Autodesk Inventor part; units mm, degrees
ref_plane "YZ Plane" through (0, 0, 0) normal (1, 0, 0) x (0, 1, 0)
ref_plane "XZ Plane" through (0, 0, 0) normal (0, 1, 0) x (-1, 0, 0)
ref_plane "XY Plane" through (0, 0, 0) normal (0, 0, 1) x (1, 0, 0)
sketch "Skizze1" plane through (0, 0, 0) normal (0, 1, 0) x (-1, 0, 0)
  circle A0 centre (32.7504, -19.9257) radius 25
  line L0 (32.7504, -19.9257) -> (-77.2496, -19.9257)
  line L1 (-77.2496, -19.9257) -> (-77.2496, -22.4257)
  line L2 (-77.2496, -22.4257) -> (7.8757, -22.4257)
  line L3 (7.8757, -22.4257) -> (7.8757, -19.9257)
  point P0 (0, 0)
  dimension "d4" = 50
  dimension "d9" = 110
  dimension "d10" = 2.5
extrude "Extrusion1" add sketch "Skizze1" along normal blind 1.5 and the other way blind 1.5 contours L3 L0 A0 | A0 L0 L3
revolve "Umdrehung1" add sketch "Skizze1" angle 360 about axis through (-32.7504, 0, -19.9257) along (1, 0, 0) picked at (7.8525, -21.3151) contours L2 L1 L0 A0 | A0 L0 L3
sketch "Skizze2" plane through (77.2496, 0, -19.9257) normal (1, 0, 0) x (0, 0, -1)
  line L0 (35, -15) -> (-35, -15)
  line L1 (-35, -15) -> (-35, 15)
  line L2 (-35, 15) -> (35, 15)
  line L3 (35, 15) -> (35, -15)
  line L4 (-25, -1.5) -> (25, 1.5)
  line L5 (35, -15) -> (-35, 15) construction
  line L6 (-35, -15) -> (35, 15) construction
  circle A0 centre (0, 0) radius 2.5
  point P0 (-19.9257, 0)
  point P1 (0, 0)
  point P2 (-3.75, 0)
  point P3 (3.75, 0)
  point P4 (-25, -1.5)
  point P5 (25, 1.5)
  dimension "d14" = 70
  dimension "d15" = 30
  dimension "d22" = 15
extrude "Extrusion2" add sketch "Skizze2" against normal blind 3 contours L0 L1 L2 L3 | A0 L4 | L4 A0
sketch "Skizze3" plane through (0, 1.5, 0) normal (0, 1, 0) x (1, 0, 0)
  line L0 (-7.8305, 17.9257) -> (-7.8757, 17.9257)
  line L1 (-7.8757, 17.9257) -> (-59.898, 17.9257)
  line L2 (-59.898, 17.9257) -> (-59.898, 68.635)
  line L3 (-59.898, 68.635) -> (-7.8757, 68.635)
  line L4 (-7.8757, 68.635) -> (-7.8757, 17.9257)
  line L5 (-7.8757, 17.9257) -> (-59.898, 17.9257)
  line L6 (-59.898, 17.9257) -> (-59.898, -26.6959)
  line L7 (-59.898, -26.6959) -> (-7.8757, -26.6959)
  line L8 (-7.8757, -26.6959) -> (-7.8757, 17.9257)
  point P0 (0, 0)
extrude "Extrusion3" cut sketch "Skizze3" against normal blind 10
properties part number "Kreisverkehrsschild_Teil_Unten"
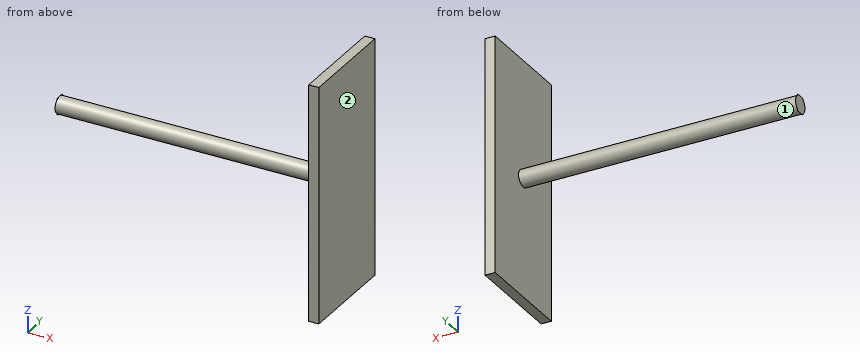
Geometry: final body of the model. Coordinates: model frame, mm. Face numbers are marked on the shaded views. Round coordinates to 2 decimals unless told otherwise and drop trailing zeros. Order: outer loops, then holes, each group sorted by start corner. A loop starts at its lowest first (then second) coordinate and runs counter-clockwise, first axis right, second up. Notation, with made-up numbers: (36, -32) - (94, -32) arc R23 cw to (94, -20) - close; hole circle Ø3 at (52, 57). An arc over 180 degrees is marked (long way). Write each question's results on one line, items separated by ' | '.
Item 1: First-contact query: pin 1 Ø4 at (y, z) = (12, -18.5) entering from -X; pin 2 Ø6 at (x, y) = (24, 4) entering from +Z; pin 3 Ø12 at (x, y) = (59.5, 5) entering from +Z. Flat tips, straight axial feed; report the tip coordinate or a pass-through.
Completed:
pin 1: x = 74.25 | pin 2: z = -17.63 | pin 3: z = -17.43
Item 2: Mould query, pull axis X, two halves, no side actions, for the marked faces 1 and 2. Classes: pulls with the +X half, pulls with the -X half, needs draft (parallel to the pull), parting line crosses it, or undercut.
Completed:
face 1: undercut | face 2: pulls with the +X half
Item 3: Section A-A, the plane z = 2.5. Return the cut outline in (x, y), and give its area (3 significant figures).
Completed:
outline: (74.25, -15) - (77.25, -15) - (77.25, 15) - (74.25, 15) - close | area: 90.0 mm^2
Item 4: Section B-B, the plane x = 12. Return the cut outline in (y, z).
Completed:
outline: circle Ø5 at (0, -19.93)
Item 5: Material intervals for line 1 along X through (y, z) = (-4.25, -34); line 2 along Z through (x, y) = (26, -1.5); line 3 along Y through (x, z) = (31, -21), sorted ascending. Write a range as [from, to].
Completed:
line 1: [74.25, 77.25] | line 2: [-21.93, -17.93] | line 3: [-2.26, 2.26]
Item 6: Section C-C, the plane y = -10. Return the cut outline in (x, z).
Completed:
outline: (74.25, -54.93) - (77.25, -54.93) - (77.25, 15.07) - (74.25, 15.07) - close
